```python
from build123d import *

# Parameters (mm, degrees)
SKETCH_1_R      = 35
SKETCH_1_R_2    = 27
EXTRUDE_1_DEPTH = 12
SKETCH_2_R      = 18
EXTRUDE_2_DEPTH = 12


with BuildPart() as part:
    # 草图1 → 凸台-拉伸1 (new body)
    with BuildSketch(Plane(origin=(0, 0, 0), x_dir=(1, 0, 0), z_dir=(0, 1, 0))):
        with Locations(Location((0, 0, 0), (0, 0, 270))):
            Circle(SKETCH_1_R)
        with Locations(Location((0, 0, 0), (0, 0, 270))):
            Circle(SKETCH_1_R_2, mode=Mode.SUBTRACT)
    extrude(amount=EXTRUDE_1_DEPTH)

    # 草图2 → 凸台-拉伸2 (add)
    with BuildSketch(Plane.XZ):
        with BuildLine():
            Line((6.363636364, 34.416625811), (59.545454545, 24.583304151))
            ThreePointArc((59.545454545, 24.583304151), (80, 0), (59.545454545, -24.583304151))
            Line((59.545454545, -24.583304151), (6.363636364, -34.416625811))
            ThreePointArc((6.363636364, -34.416625811), (35, 0), (6.363636364, 34.416625811))
        make_face()
        with Locations(Location((55, 0, 0), (0, 0, 270))):
            Circle(SKETCH_2_R, mode=Mode.SUBTRACT)
    extrude(amount=-EXTRUDE_2_DEPTH)


solid = part.part
```
Part model, mm, in its own coordinate system. Coordinates: 2 decimals unless noted, no trailing zeros. Order: outer loops, then holes, each group sorted by start corner. A loop starts at its lowest first (then second) coordinate and runs counter-clockwise, first axis right, second up. Notation, with made-up numbers: (-38.5, 4) -> (3.5, 4) arc R33 ccw to (3.5, 32) -> close; hole circle Ø5 at (-6, 72.25). An arc over 180 degrees is marked (long way). Put each result on its own line as item: value. Start each with the question number.
(1) Band-saw the part on B-B (y = 10). Give the cut face in (x, z).
(2) Band-saw the part on A-A (z = 0). Give the cut face in (x, y), then the cut area to 3 significant figures.
(3) Mould opens along Z. For faces 1 (the face through (70.178, 5.916, -9.677)), 2 (the face through (80, 6, 0)), 3 (the face through (33.33, 5.92, -29.43)), 4 (the face through (23, 0, 15)) say: pulls with the +Z half, pulls with the -Z half, needs draft (parallel to the pull), parting line crosses it, or undercut.
(4) Probe line 1 along X through (y, z) = (8.75, 0); line 2 along X through (y, z) = (11, -14); line 3 along Z through (x, y) = (49, 10.5). List the from-to ranges inside material, lowest first. Write a range as [from, to].
(5) Band-saw the part on C-C (x = 0). Give the cut face in (y, z), then the cut area to 3 significant figures.
(6) Band-saw the part on D-D (x = 55). Give the cut face in (y, z), then the cut area to 3 significant figures.
(7) Pin check, flat tips, straight feed: pin 1 Ø3 at (y, z) = (9.5, -17.5) entering from -X; pin 2 Ø1 at (x, y) = (39, 9.5) entering from +Z; pin 3 Ø6 at (y, z) = (3.5, -24.5) entering from -X; pin 4 Ø21.5 at (x, z) = (55, 0) entering from +Y. Stop position of each tip, or through.
Determined:
1. outline: (6.36, -34.42) -> (59.55, -24.58) arc R25 ccw to (59.55, 24.58) -> (6.36, 34.42) arc R35 ccw (long way) to start; hole circle Ø54 at (0, 0); hole circle Ø36 at (55, 0)
2. outline: (-35, 0) -> (-27, 0) -> (-27, 12) -> (-35, 12) -> close; (27, 0) -> (37, 0) -> (37, 12) -> (27, 12) -> close; (73, 0) -> (80, 0) -> (80, 12) -> (73, 12) -> close
2. area: 300 mm²
3. face 1: undercut
3. face 2: parting line crosses it
3. face 3: pulls with the -Z half
3. face 4: needs draft
4. line 1: x = [-35, -27], [27, 37], [73, 80]
4. line 2: x = [-32.08, -23.09], [23.09, 43.69], [66.31, 75.71]
4. line 3: z = [-26.53, -16.97], [16.97, 26.53]
5. outline: (0, -35) -> (12, -35) -> (12, -27) -> (0, -27) -> close; (0, 27) -> (12, 27) -> (12, 35) -> (0, 35) -> close
5. area: 192 mm²
6. outline: (0, -25.42) -> (12, -25.42) -> (12, -18) -> (0, -18) -> close; (0, 18) -> (12, 18) -> (12, 25.42) -> (0, 25.42) -> close
6. area: 178 mm²
7. pin 1: stops at x = -31.13
7. pin 2: stops at z = 28.47
7. pin 3: stops at x = -27.62
7. pin 4: passes through
